Read the model definition and answer for the solid it produces. Units are mm, in the model's axes. A direction names the side the tool comes from. Round coordinates to 2 decimals unless told otherwise and drop trailing zeros. Order: outer loops, then holes, each group sorted by start corner. A loop starts at its lowest first (then second) coordinate and runs counter-clockwise, first axis right, second up. Notation, with made-up numbers: (81.25, 75) -> (112.25, 75) arc R34 ccw to (112.25, 110) -> close; hole circle Ø5 at (56.5, 51.5). An arc over 180 degrees is marked (long way). Answer as a JSON object with one key per item and string values. Group by question number.
Item 1: The mould has two halves that part along X. Classify faces 1 (the flat face through (87, 8, 8)), 2 (the flat face through (27, 1, 52)), 3 (the flat face through (83, 1, 8)): pulls with the +X half, pulls with the -X half, needs draft (parallel to the pull), parting line crosses it, or undercut.
Item 2: Section A-A, the plane x = 61.5 is taken. Write down the section's boundary in (y, z).
Item 3: For faces 4 (the flat face through (38.5, 4, 52)), 5 (the flat face through (3, 4, 26)), 6 (the flat face through (32, 4.7, 57)), determine the directions among +Z, -Z, +X, -X, +Y, -Y from which every point of the face is accessible in a straight line to the end or side of a thin tool.
Item 4: Given P1, Ø4.5, axis at x = 9.5, z = 54.5, coming from the -Y side; P2, Ø0.6, axis at x = 85.5, z = 28, coming from the -Y side; P3, Ø4, axis at x = 60.5, y = 4.5, coming from the +Z side; P4, Ø0.8, axis at x = 28.5, z = 2.5, coming from the +Y side, each flat-ended and moving along its own axis, determine where each tip first touches the part or whether it passes through.
Item 5: Consider probe 1 along Z at (x, y) = (61.5, -0.55); probe 2 along Y at (x, z) = (82.5, 4); probe 3 along Y at (x, z) = (26.5, 46.5). Determine where each line is inside the solid, lowest interval first. Write a range as from..to.
from build123d import *

# Parameters (mm, degrees)
SKETCH_W        = 85
SKETCH_H        = 56
SKETCH_R        = 1.5
PAD_DEPTH       = 1.5
SKETCH001_W     = 17
SKETCH001_H     = 12
PAD001_DEPTH    = 16
SKETCH002_W     = 9
SKETCH002_H     = 5
POCKET_DEPTH    = 9
SKETCH003_W     = 21
SKETCH003_H     = 16
PAD002_DEPTH    = 13
SKETCH004_W     = 13
SKETCH004_H     = 10
POCKET001_DEPTH = 10
SKETCH005_W     = 14
SKETCH005_H     = 12
PAD003_DEPTH    = 5
POCKET002_DEPTH = 12
POCKET003_DEPTH = 10
SKETCH008_W     = 7
SKETCH008_H     = 5
PAD004_DEPTH    = 3
POCKET004_DEPTH = 5
POCKET005_DEPTH = 4
SKETCH011_W     = 6
SKETCH011_H     = 12
PAD005_DEPTH    = 5
SKETCH012_R     = 2
PAD006_DEPTH    = 2
SKETCH013_R     = 1.5
POCKET006_DEPTH = 10
SKETCH014_W     = 50
SKETCH014_H     = 5
PAD007_DEPTH    = 1.5
SKETCH015_R     = 0.5
PAD008_DEPTH    = 6
SKETCH016_W     = 2
SKETCH016_H     = 22
PAD009_DEPTH    = 4
SKETCH017_W     = 15
SKETCH017_H     = 15
SKETCH017_W_2   = 8
SKETCH017_H_2   = 8
PAD010_DEPTH    = 1.5
SKETCH018_W     = 13
SKETCH018_H     = 13
PAD011_DEPTH    = 1.5


with BuildPart() as part:
    # Sketch → Pad (new body)
    with BuildSketch(Plane.XZ):
        with Locations((42.5, 28)):
            Rectangle(SKETCH_W, SKETCH_H)
        with Locations((3.5, 52.5)):
            Circle(SKETCH_R, mode=Mode.SUBTRACT)
        with Locations((61.5, 52.5)):
            Circle(SKETCH_R, mode=Mode.SUBTRACT)
        with Locations((61.5, 3.5)):
            Circle(SKETCH_R, mode=Mode.SUBTRACT)
        with Locations((3.5, 3.5)):
            Circle(SKETCH_R, mode=Mode.SUBTRACT)
    extrude(amount=PAD_DEPTH)

    # Sketch001 (on Face9 of Pad) → Pad001 (join)
    with BuildSketch(Plane(origin=(0, 0, 0), x_dir=(1, 0, 0), z_dir=(0, 1, 0))):
        with Locations((78.5, -8)):
            Rectangle(SKETCH001_W, SKETCH001_H)
        with Locations((78.5, -25)):
            Rectangle(SKETCH001_W, SKETCH001_H)
    extrude(amount=PAD001_DEPTH)

    # Sketch002 (on Face19 of Pad001) → Pocket (cut)
    with BuildSketch(Plane(origin=(87, 0, 0), x_dir=(0, 0, 1), z_dir=(1, 0, 0))):
        with Locations((8, -3.5)):
            Rectangle(SKETCH002_W, SKETCH002_H)
        with Locations((8, -12.5)):
            Rectangle(SKETCH002_W, SKETCH002_H)
        with Locations((25, -3.5)):
            Rectangle(SKETCH002_W, SKETCH002_H)
        with Locations((25, -12.5)):
            Rectangle(SKETCH002_W, SKETCH002_H)
    extrude(amount=-POCKET_DEPTH, mode=Mode.SUBTRACT)

    # Sketch003 (on Face4 of Pocket) → Pad002 (join)
    with BuildSketch(Plane(origin=(0, 0, 0), x_dir=(1, 0, 0), z_dir=(0, 1, 0))):
        with Locations((76.5, -46)):
            Rectangle(SKETCH003_W, SKETCH003_H)
    extrude(amount=PAD002_DEPTH)

    # Sketch004 (on Face25 of Pad002) → Pocket001 (cut)
    with BuildSketch(Plane(origin=(87, 0, 0), x_dir=(0, 0, 1), z_dir=(1, 0, 0))):
        with Locations((46, -6)):
            Rectangle(SKETCH004_W, SKETCH004_H)
    extrude(amount=-POCKET001_DEPTH, mode=Mode.SUBTRACT)

    # Sketch005 (on Face4 of Pocket001) → Pad003 (join)
    with BuildSketch(Plane(origin=(0, 0, 0), x_dir=(1, 0, 0), z_dir=(0, 1, 0))):
        with Locations((32, -51)):
            Rectangle(SKETCH005_W, SKETCH005_H)
    extrude(amount=PAD003_DEPTH)

    # Sketch006 (on Face33 of Pad003) → Pocket002 (cut)
    with BuildSketch(Plane(origin=(0, 0, 57), x_dir=(-1, 0, 0), z_dir=(0, 0, 1))):
        Polygon((-39, 0), (-37, 0), (-39, -2), align=None)
        Polygon((-27, 0), (-25, 0), (-25, -2), align=None)
    extrude(amount=-POCKET002_DEPTH, mode=Mode.SUBTRACT)

    # Sketch007 (on Face38 of Pocket002) → Pocket003 (cut)
    with BuildSketch(Plane(origin=(0, 0, 57), x_dir=(-1, 0, 0), z_dir=(0, 0, 1))):
        Polygon((-25.5, -2.5), (-25.5, -4.5), (-38.5, -4.5), (-38.5, -2.5), (-36.5, -0.5), (-27.5, -0.5), align=None)
    extrude(amount=-POCKET003_DEPTH, mode=Mode.SUBTRACT)

    # Sketch008 (on Face4 of Pocket003) → Pad004 (join)
    with BuildSketch(Plane(origin=(0, 0, 0), x_dir=(1, 0, 0), z_dir=(0, 1, 0))):
        with Locations((10.5, -54.5)):
            Rectangle(SKETCH008_W, SKETCH008_H)
    extrude(amount=PAD004_DEPTH)

    # Sketch009 (on Face37 of Pad004) → Pocket004 (cut)
    with BuildSketch(Plane(origin=(0, 0, 57), x_dir=(-1, 0, 0), z_dir=(0, 0, 1))):
        Polygon((-14, 0), (-12.91, 0), (-14, -1), align=None)
        Polygon((-8, 0), (-7, 0), (-7, -1), align=None)
    extrude(amount=-POCKET004_DEPTH, mode=Mode.SUBTRACT)

    # Sketch010 (on Face48 of Pocket004) → Pocket005 (cut)
    with BuildSketch(Plane(origin=(0, 0, 57), x_dir=(-1, 0, 0), z_dir=(0, 0, 1))):
        Polygon((-7.5, -1.5), (-7.5, -2.5), (-13.5, -2.5), (-13.5, -1.5), (-12.5, -0.5), (-8.5, -0.5), align=None)
    extrude(amount=-POCKET005_DEPTH, mode=Mode.SUBTRACT)

    # Sketch011 (on Face4 of Pocket005) → Pad005 (join)
    with BuildSketch(Plane(origin=(0, 0, 0), x_dir=(1, 0, 0), z_dir=(0, 1, 0))):
        with Locations((53, -50)):
            Rectangle(SKETCH011_W, SKETCH011_H)
    extrude(amount=PAD005_DEPTH)

    # Sketch012 (on Face32 of Pad005) → Pad006 (join)
    with BuildSketch(Plane(origin=(0, 0, 56), x_dir=(-1, 0, 0), z_dir=(0, 0, 1))):
        with Locations((-53, -2.5)):
            Circle(SKETCH012_R)
    extrude(amount=PAD006_DEPTH)

    # Sketch013 (on Face75 of Pad006) → Pocket006 (cut)
    with BuildSketch(Plane(origin=(0, 0, 58), x_dir=(-1, 0, 0), z_dir=(0, 0, 1))):
        with Locations((-53, -2.5)):
            Circle(SKETCH013_R)
    extrude(amount=-POCKET006_DEPTH, mode=Mode.SUBTRACT)

    # Sketch014 (on Face4 of Pocket006) → Pad007 (join)
    with BuildSketch(Plane(origin=(0, 0, 0), x_dir=(1, 0, 0), z_dir=(0, 1, 0))):
        with Locations((32, -3.5)):
            Rectangle(SKETCH014_W, SKETCH014_H)
    extrude(amount=PAD007_DEPTH)

    # Sketch015 (on Face56 of Pad007) → Pad008 (join)
    with BuildSketch(Plane(origin=(0, 1.5, 0), x_dir=(1, 0, 0), z_dir=(0, 1, 0))):
        with Locations((8, -4.79)):
            Circle(SKETCH015_R)
        with Locations((10.54, -4.79)):
            Circle(SKETCH015_R)
        with Locations((13.08, -4.79)):
            Circle(SKETCH015_R)
        with Locations((15.62, -4.79)):
            Circle(SKETCH015_R)
        with Locations((18.16, -4.79)):
            Circle(SKETCH015_R)
        with Locations((20.7, -4.79)):
            Circle(SKETCH015_R)
        with Locations((23.24, -4.79)):
            Circle(SKETCH015_R)
        with Locations((25.78, -4.79)):
            Circle(SKETCH015_R)
        with Locations((28.32, -4.79)):
            Circle(SKETCH015_R)
        with Locations((30.86, -4.79)):
            Circle(SKETCH015_R)
        with Locations((8, -2.25)):
            Circle(SKETCH015_R)
        with Locations((10.54, -2.25)):
            Circle(SKETCH015_R)
        with Locations((13.08, -2.25)):
            Circle(SKETCH015_R)
        with Locations((15.62, -2.25)):
            Circle(SKETCH015_R)
        with Locations((18.16, -2.25)):
            Circle(SKETCH015_R)
        with Locations((20.7, -2.25)):
            Circle(SKETCH015_R)
        with Locations((23.24, -2.25)):
            Circle(SKETCH015_R)
        with Locations((25.78, -2.25)):
            Circle(SKETCH015_R)
        with Locations((28.32, -2.25)):
            Circle(SKETCH015_R)
        with Locations((30.86, -2.25)):
            Circle(SKETCH015_R)
        with Locations((33.4, -2.25)):
            Circle(SKETCH015_R)
        with Locations((33.4, -4.79)):
            Circle(SKETCH015_R)
        with Locations((35.94, -2.25)):
            Circle(SKETCH015_R)
        with Locations((35.94, -4.79)):
            Circle(SKETCH015_R)
        with Locations((38.48, -2.25)):
            Circle(SKETCH015_R)
        with Locations((38.48, -4.79)):
            Circle(SKETCH015_R)
        with Locations((41.02, -2.25)):
            Circle(SKETCH015_R)
        with Locations((41.02, -4.79)):
            Circle(SKETCH015_R)
        with Locations((43.56, -2.25)):
            Circle(SKETCH015_R)
        with Locations((43.56, -4.79)):
            Circle(SKETCH015_R)
        with Locations((46.1, -2.25)):
            Circle(SKETCH015_R)
        with Locations((48.64, -2.25)):
            Circle(SKETCH015_R)
        with Locations((51.18, -2.25)):
            Circle(SKETCH015_R)
        with Locations((53.72, -2.25)):
            Circle(SKETCH015_R)
        with Locations((56.26, -2.25)):
            Circle(SKETCH015_R)
        with Locations((46.1, -4.79)):
            Circle(SKETCH015_R)
        with Locations((48.64, -4.79)):
            Circle(SKETCH015_R)
        with Locations((51.18, -4.79)):
            Circle(SKETCH015_R)
        with Locations((53.72, -4.79)):
            Circle(SKETCH015_R)
        with Locations((56.26, -4.79)):
            Circle(SKETCH015_R)
    extrude(amount=PAD008_DEPTH)

    # Sketch016 (on Face4 of Pad008) → Pad009 (join)
    with BuildSketch(Plane(origin=(0, 0, 0), x_dir=(1, 0, 0), z_dir=(0, 1, 0))):
        with Locations((3, -26)):
            Rectangle(SKETCH016_W, SKETCH016_H)
        with Locations((44, -43)):
            Rectangle(SKETCH016_W, SKETCH016_H)
    extrude(amount=PAD009_DEPTH)

    # Sketch017 (on Face4 of Pad009) → Pad010 (join)
    with BuildSketch(Plane(origin=(0, 0, 0), x_dir=(1, 0, 0), z_dir=(0, 1, 0))):
        with Locations((22.5, -23.5)):
            Rectangle(SKETCH017_W, SKETCH017_H)
        with Locations((59, -21)):
            Rectangle(SKETCH017_W_2, SKETCH017_H_2)
    extrude(amount=PAD010_DEPTH)

    # Sketch018 (on Face5 of Pad010) → Pad011 (join)
    with BuildSketch(Plane.XZ.offset(1.5)):
        with Locations((45.5, 23.5)):
            Rectangle(SKETCH018_W, SKETCH018_H)
    extrude(amount=PAD011_DEPTH)


solid = part.part
Values found:
{
 "1": {"face 1": "pulls with the +X half", "face 2": "undercut", "face 3": "needs draft"},
 "2": {"outline": "(-1.5, 0) -> (0, 0) -> (0, 2) -> (-1.5, 2) -> close; (-1.5, 5) -> (0, 5) -> (0, 17) -> (1.5, 17) -> (1.5, 25) -> (0, 25) -> (0, 51) -> (-1.5, 51) -> close; (-1.5, 54) -> (0, 54) -> (0, 56) -> (-1.5, 56) -> close"},
 "3": {"face 4": "+Z", "face 5": "+Z, -Z, -X, +Y", "face 6": "+Z, -X, +Y, -Y"},
 "4": {"P1": "y = -1.5", "P2": "y = 0", "P3": "through", "P4": "y = 7.5"},
 "5": {"probe 1": "0..2, 5..51, 54..56", "probe 2": "-1.5..1, 6..10, 15..16", "probe 3": "-1.5..0, 0.5..5"}
}
